Could you check a few things on this model? Use its own coordinates, in mm. Face numbers are marked on the shaded views. A direction names the side the tool comes from. Coordinates: 2 decimals unless noted, no trailing zeros. Order: outer loops, then holes, each group sorted by start corner. A loop starts at its lowest first (then second) coordinate and runs counter-clockwise, first axis right, second up.
```python
from build123d import *

# Parameters (mm, degrees)
F3_W     = 14.3
F3_H     = 18.15
F4_DEPTH = 7.6
F5_R     = 0.5
F0_T     = 0.5
F2_D     = 1.1


# Not quite as in the source:
# - a shell that OpenCascade refuses in one call is made with other operations: the cavity is built on its own and cut out


with BuildPart() as f4:
    # F3 (on Top) → F4 (new body)
    with BuildSketch(Plane.XY):
        Rectangle(F3_W, F3_H)
    extrude(amount=F4_DEPTH)

    # F5
    f5_edges = [f4.edges().sort_by_distance(p)[0] for p in [
        (-7.15, -9.075, 3.8),
        (7.15, -9.075, 3.8),
        (7.15, 0, 7.6),
        (-7.15, 9.075, 3.8),
        (7.15, 9.075, 3.8),
        (-7.15, 0, 7.6),
        (0, 9.075, 7.6),
        (0, -9.075, 7.6),
    ]]
    fillet(f5_edges, radius=F5_R)

    # F0: shell of thickness 0.5, made by hand


with BuildPart() as f0_core1:
    # F0_t2: copy of F4
    add(f4.part)

    # the walls: a layer under each face that stays
    f0_faces = [f0_core1.faces().sort_by_distance(p)[0] for p in [
        (0, -9.075, 3.55),
        (-7.15, 0, 3.55),
        (7.15, 0, 3.55),
        (0, 9.075, 3.55),
        (0, 0, 7.6),
    ]]
    thicken(f0_faces, amount=-F0_T, mode=Mode.SUBTRACT)


with BuildPart() as f4_1:
    add(f4.part)

    # what is left inside the walls is the cavity
    f0_cavity = [f0_core1.part.solids().sort_by_distance(p)[0] for p in [
        (0, -2.858333, 0.005),
    ]]
    add(f0_cavity, mode=Mode.SUBTRACT)

    # F2 (through all)
    with Locations(Plane.XY.offset(7.6)):
        with Locations((0, 4.4)):
            Hole(F2_D / 2)


solid = f4_1.part
```
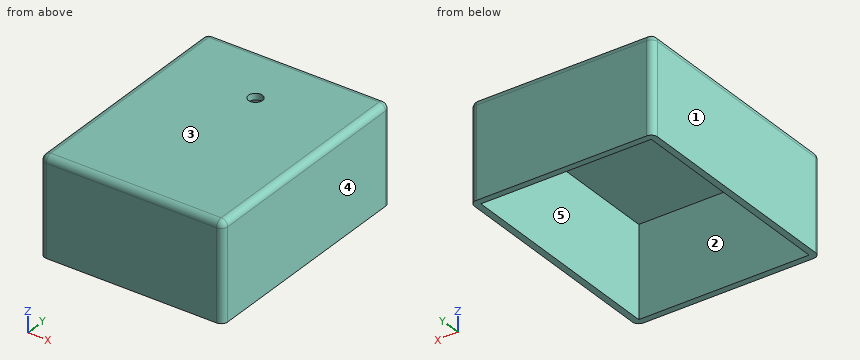
Item 1: For pin 1 Ø4 at (x, y) = (-1, -2) entering from -Z; pin 2 Ø1.3 at (x, y) = (0, 4.4) entering from +Z, each with a flat end and sliding along its axis, tell me the tip position at first contact or that it passes through.
Item 2: I need wall thicknesses on line 1 (Y direction, x = 3, z = 4) (3 decimals); line 2 (X direction, y = 1, z = 5.5). Which ranges of each line are inside material? Lowest first, please.
Item 3: Suppose I cut it at D-D (y = -5.25). List the corners of the cut face in (x, z) for me, and give its area (3 significant figures).
Item 4: Thinking about a two-plate mould opening in X: for the marked faces 1, 2 and 3, which applies, +X half, -X half, draft (parallel to the pull), parting line (faces both ways), or undercut?
Item 5: Suppose I cut it at B-B (z = 5). List the corners of the cut face in (x, y) for me (3 decimals).
Item 6: Suppose I cut it at C-C (y = 4.4). List the corners of the cut face in (x, z) for me, and give its area (3 significant figures).
Item 7: Suppose I cut it at A-A (x = 0). List the corners of the cut face in (y, z) for me (3 decimals).
Item 8: Which directions (+Z, -Z, +X, -X, +Y, -Y) give clear straight access to the entire face, cutting with the end or side of a thin tool? Please do the marked faces 4 and 5.
Geometry results:
1. pin 1: stops at z = 7.1
1. pin 2: stops at z = 7.6
2. line 1: y = -9.075 to -8.575, 8.575 to 9.075
2. line 2: x = -7.15 to -6.65, 6.65 to 7.15
3. outline: (-7.15, 0) - (-6.65, 0) - (-6.65, 7.1) - (6.65, 7.1) - (6.65, 0) - (7.15, 0) - (7.15, 7.1) arc R0.5 ccw to (6.65, 7.6) - (-6.65, 7.6) arc R0.5 ccw to (-7.15, 7.1) - close
3. area: 14.1 mm2
4. face 1: -X half
4. face 2: undercut
4. face 3: draft
5. outline: (-7.15, -8.575) arc R0.5 ccw to (-6.65, -9.075) - (6.65, -9.075) arc R0.5 ccw to (7.15, -8.575) - (7.15, 8.575) arc R0.5 ccw to (6.65, 9.075) - (-6.65, 9.075) arc R0.5 ccw to (-7.15, 8.575) - close; hole (-6.65, -8.575) - (6.65, -8.575) - (6.65, 8.575) - (-6.65, 8.575) - close
6. outline: (-7.15, 0) - (-6.65, 0) - (-6.65, 7.1) - (-0.55, 7.1) - (-0.55, 7.6) - (-6.65, 7.6) arc R0.5 ccw to (-7.15, 7.1) - close; (0.55, 7.1) - (6.65, 7.1) - (6.65, 0) - (7.15, 0) - (7.15, 7.1) arc R0.5 ccw to (6.65, 7.6) - (0.55, 7.6) - close
6. area: 13.6 mm2
7. outline: (-9.075, 0) - (-8.575, 0) - (-8.575, 7.1) - (3.85, 7.1) - (3.85, 7.6) - (-8.575, 7.6) arc R0.5 ccw to (-9.075, 7.1) - close; (4.95, 7.1) - (8.575, 7.1) - (8.575, 0) - (9.075, 0) - (9.075, 7.1) arc R0.5 ccw to (8.575, 7.6) - (4.95, 7.6) - close
8. face 4: +Z, -Z, +X, +Y, -Y
8. face 5: -Z
